Geometry check sheet. Reference: the model listing, model coordinates, mm. Face numbers are marked on the shaded views. A direction names the side the tool comes from. Round coordinates to 2 decimals unless told otherwise and drop trailing zeros. Loops run counter-clockwise (first coordinate to the right, second up) from the corner with the lowest first, then second, coordinate; pieces in that order, holes last. Notation, with made-up numbers: (-3, 79.25) -> (7, 79.25) arc R18 ccw to (7, 105.25) -> close; hole circle Ø11 at (45.5, 54). An arc over 180 degrees is marked (long way). Use a Markdown table: item, result. Add a question column.
Q1. Sectioned sample at B-B, the plane y = -6.25. Enter the section's corners in (x, z), then the cut area to 4 significant figures.
Q2. Set-up check for the marked faces 4, 5, 6 and 7: record each of +Z, -Z, +X, -X, +Y, -Y from which the full face is reachable in a straight line by a thin tool's end or side.
Q3. Sectioned sample at A-A, the plane x = 29.5. Enter the section's corners in (y, z), then the cut area to 3 significant figures.
Q4. Sectioned sample at D-D, the plane x = -42. Enter the section's corners in (y, z), then the cut area to 3 significant figures.
Q5. Release check for a two-part mould opening along X. For the marked faces 1, 2 and 3 record: released by +X, released by -X, zero draft, split by the parting line, or undercut.
Q6. Gauge pin test, flat ends, axial feed: P1, Ø2, axis at x = -1, z = 2.5, coming from the +Y side; P2, Ø2, axis at x = -10, y = 5.5, coming from the +Z side; P3, Ø2, axis at x = 17, y = 5, coming from the -Z side. Record the tip position at first contact, or that the pin passes through.
Q7. Sectioned sample at C-C, the plane z = -24. Enter the section's corners in (x, y).
Q8. Material ranges on L1, parallel to Z at x = -17, y = -0.1; L2, parallel to X at y = -4.25, z = -20.5; L3, parallel to Z at x = -13.5, y = 6.75, recorded low to high.
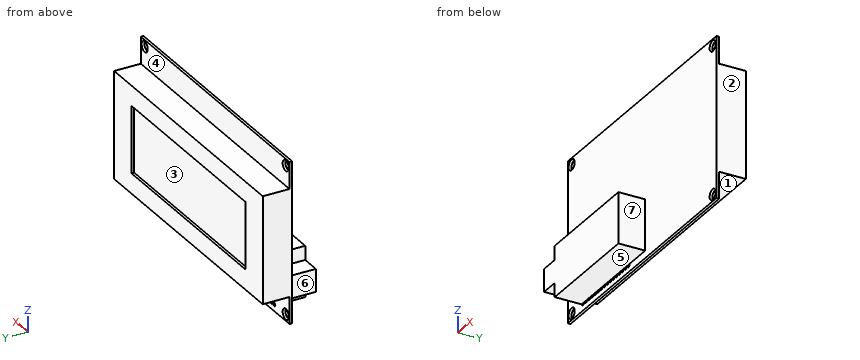
```python
from build123d import *

# Parameters (mm, degrees)
ESQUISSE1_W             = 98
ESQUISSE1_H             = 60
ESQUISSE1_R             = 2
ESQUISSE1_R_2           = 0.637876667
BOSS_EXTRU_1_DEPTH      = 0.5
ESQUISSE3_W             = 98
ESQUISSE3_H             = 40
BOSS_EXTRU_2_DEPTH      = 10
ESQUISSE4_W             = 75
ESQUISSE4_H             = 25
ENL_V_MAT_EXTRU_1_DEPTH = 1
BOSS_EXTRU_4_DEPTH      = 10


with BuildPart() as part:
    # Esquisse1 → Boss.-Extru.1 (new, symmetric)
    with BuildSketch(Plane(origin=(0, 0, 0), x_dir=(1, 0, 0), z_dir=(0, 1, 0))):
        Rectangle(ESQUISSE1_W, ESQUISSE1_H)
        with Locations(Location((-46.5, 27.5, 0), (0, 0, 270))):
            Circle(ESQUISSE1_R, mode=Mode.SUBTRACT)
        with Locations(Location((46.5, 27.5, 0), (0, 0, 90))):
            Circle(ESQUISSE1_R, mode=Mode.SUBTRACT)
        with Locations(Location((46.5, -27.5, 0), (0, 0, 270))):
            Circle(ESQUISSE1_R, mode=Mode.SUBTRACT)
        with Locations(Location((-46.5, -27.5, 0), (0, 0, 90))):
            Circle(ESQUISSE1_R, mode=Mode.SUBTRACT)
        with Locations(Location((-39, 27.5, 0), (0, 0, 270))):
            Circle(ESQUISSE1_R_2, mode=Mode.SUBTRACT)
        with Locations(Location((-37, 27.5, 0), (0, 0, 270))):
            Circle(ESQUISSE1_R_2, mode=Mode.SUBTRACT)
        with Locations(Location((-35, 27.5, 0), (0, 0, 270))):
            Circle(ESQUISSE1_R_2, mode=Mode.SUBTRACT)
        with Locations(Location((-33, 27.5, 0), (0, 0, 270))):
            Circle(ESQUISSE1_R_2, mode=Mode.SUBTRACT)
        with Locations(Location((-31, 27.5, 0), (0, 0, 270))):
            Circle(ESQUISSE1_R_2, mode=Mode.SUBTRACT)
        with Locations(Location((-29, 27.5, 0), (0, 0, 270))):
            Circle(ESQUISSE1_R_2, mode=Mode.SUBTRACT)
        with Locations(Location((-27, 27.5, 0), (0, 0, 270))):
            Circle(ESQUISSE1_R_2, mode=Mode.SUBTRACT)
        with Locations(Location((-25, 27.5, 0), (0, 0, 270))):
            Circle(ESQUISSE1_R_2, mode=Mode.SUBTRACT)
        with Locations(Location((-23, 27.5, 0), (0, 0, 270))):
            Circle(ESQUISSE1_R_2, mode=Mode.SUBTRACT)
        with Locations(Location((-21, 27.5, 0), (0, 0, 270))):
            Circle(ESQUISSE1_R_2, mode=Mode.SUBTRACT)
        with Locations(Location((-19, 27.5, 0), (0, 0, 270))):
            Circle(ESQUISSE1_R_2, mode=Mode.SUBTRACT)
        with Locations(Location((-17, 27.5, 0), (0, 0, 270))):
            Circle(ESQUISSE1_R_2, mode=Mode.SUBTRACT)
        with Locations(Location((-15, 27.5, 0), (0, 0, 270))):
            Circle(ESQUISSE1_R_2, mode=Mode.SUBTRACT)
        with Locations(Location((-13, 27.5, 0), (0, 0, 270))):
            Circle(ESQUISSE1_R_2, mode=Mode.SUBTRACT)
        with Locations(Location((-11, 27.5, 0), (0, 0, 270))):
            Circle(ESQUISSE1_R_2, mode=Mode.SUBTRACT)
        with Locations(Location((-9, 27.5, 0), (0, 0, 270))):
            Circle(ESQUISSE1_R_2, mode=Mode.SUBTRACT)
    extrude(amount=BOSS_EXTRU_1_DEPTH, both=True)

    # Esquisse3 → Boss.-Extru.2 (add)
    with BuildSketch(Plane(origin=(0, 0.5, 0), x_dir=(1, 0, 0), z_dir=(0, 1, 0))):
        Rectangle(ESQUISSE3_W, ESQUISSE3_H)
    extrude(amount=BOSS_EXTRU_2_DEPTH)

    # Esquisse4 → Enlèv. mat.-Extru.1 (cut)
    with BuildSketch(Plane(origin=(0, 10.5, 0), x_dir=(1, 0, 0), z_dir=(0, 1, 0))):
        Rectangle(ESQUISSE4_W, ESQUISSE4_H)
    extrude(amount=-ENL_V_MAT_EXTRU_1_DEPTH, mode=Mode.SUBTRACT)

    # Esquisse5 → Boss.-Extru.4 (add)
    with BuildSketch(Plane.XZ.offset(0.5)):
        Polygon((-40, -27.25), (-40, -22), (-47, -22), (-47, -13.5), (-40, -13.5), (-40, -8.25), (2, -8.25), (2, -27.25), align=None)
    extrude(amount=BOSS_EXTRU_4_DEPTH)


solid = part.part
```
Values:
| question | item | result |
|---|---|---|
| 1 | outline | (-47, -22) -> (-40, -22) -> (-40, -27.25) -> (2, -27.25) -> (2, -8.25) -> (-40, -8.25) -> (-40, -13.5) -> (-47, -13.5) -> close |
| 1 | area | 857.5 mm^2 |
| 2 | face 4 | +Z, +X, -X, +Y |
| 2 | face 5 | -Z, +X, -X, -Y |
| 2 | face 6 | +Z, -Z, -X, -Y |
| 2 | face 7 | +Z, -Z, +X, -Y |
| 3 | outline | (-0.5, -30) -> (0.5, -30) -> (0.5, -20) -> (10.5, -20) -> (10.5, -12.5) -> (9.5, -12.5) -> (9.5, 12.5) -> (10.5, 12.5) -> (10.5, 20) -> (0.5, 20) -> (0.5, 30) -> (-0.5, 30) -> close |
| 3 | area | 435 mm^2 |
| 4 | outline | (-10.5, -22) -> (-0.5, -22) -> (-0.5, -30) -> (0.5, -30) -> (0.5, -20) -> (10.5, -20) -> (10.5, 20) -> (0.5, 20) -> (0.5, 30) -> (-0.5, 30) -> (-0.5, -13.5) -> (-10.5, -13.5) -> close |
| 4 | area | 545 mm^2 |
| 5 | face 1 | zero draft |
| 5 | face 2 | released by +X |
| 5 | face 3 | undercut |
| 6 | P1 | y = 9.5 |
| 6 | P2 | z = 20 |
| 6 | P3 | z = -20 |
| 7 | outline | (-49, -0.5) -> (-40, -0.5) -> (-40, -10.5) -> (2, -10.5) -> (2, -0.5) -> (49, -0.5) -> (49, 0.5) -> (-49, 0.5) -> close |
| 8 | L1 | -30 to -28.14, -26.86 to 30 |
| 8 | L2 | -47 to 2 |
| 8 | L3 | -20 to 20 |
